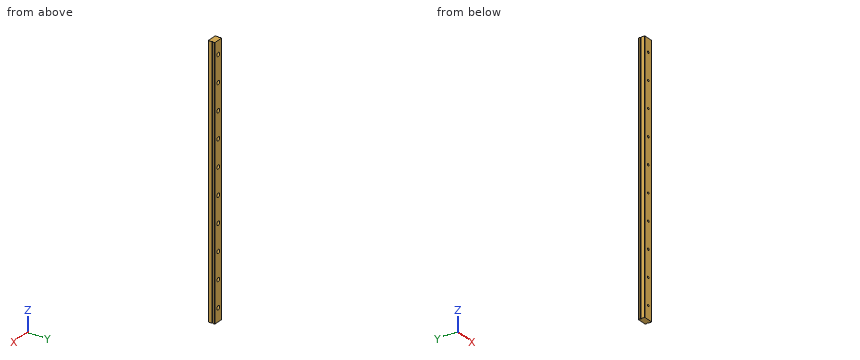
from build123d import *

# Parameters (mm, degrees)
EXTRUDE_1_DEPTH           = 400
HOLE_WIZARD_2_D           = 3.2
HOLE_WIZARD_2_CBORE_D     = 6
HOLE_WIZARD_2_CBORE_DEPTH = 4.5


with BuildPart() as part:
    # 草图1 → 凸台-拉伸1 (new body)
    with BuildSketch(Plane.XY):
        Polygon((-3.269035533, 4.949238579), (10.730964467, 4.949238579), (11.230964467, 4.449238579), (11.230964467, 2.317517259), (10.086764657, 1.783377919), (10.086764657, 0.983377919), (11.230964467, 0.449238579), (11.230964467, -4.550761421), (10.730964467, -5.050761421), (-3.269035533, -5.050761421), (-3.769035533, -4.550761421), (-3.769035533, 0.449238579), (-2.624835723, 0.983377919), (-2.624835723, 1.783377919), (-3.769035533, 2.317517259), (-3.769035533, 4.449238579), align=None)
    extrude(amount=-EXTRUDE_1_DEPTH)

    # 孔2 (through all)
    with Locations(Plane(origin=(3.730964467, 4.949238579, -380), x_dir=(0, 0, 1), z_dir=(0, 1, 0))):
        with Locations((0, 0), (40, 0), (80, 0), (120, 0), (160, 0), (200, 0), (240, 0), (280, 0), (320, 0), (360, 0)):
            CounterBoreHole(HOLE_WIZARD_2_D / 2, HOLE_WIZARD_2_CBORE_D / 2, HOLE_WIZARD_2_CBORE_DEPTH)


solid = part.part
Source: CAD feature listing. Evaluate the final solid. Frame: model axes, mm. Coordinates: 2 decimals unless noted, no trailing zeros. Write each loop counter-clockwise with the first axis right and the second up, starting at its lowest first coordinate (ties: lowest second). Pieces come first, ordered by that corner, then holes. Notation, with made-up numbers: M 81.5,11 L 89.5,11 A26 cw 89.5,33 Z; hole C -34,8.5 d8. An arc over 180 degrees is marked long. Use a Markdown table: item, result.
1) First-contact query: pin 1 Ø2.5 at (x, z) = (3.73, -380) entering from -Y; pin 2 Ø3 at (x, z) = (4.5, -259.5) entering from +Y. Flat tips, straight axial feed; report the tip coordinate or a pass-through.
Conclusion:
| item | result |
|---|---|
| pin 1 | passes through |
| pin 2 | stops at y = 0.45 |
2) Ray query, L1, parallel to X at y = -3.15, z = -380; L2, parallel to X at y = 2.3, z = -60; L3, parallel to X at y = 4.5, z = -248. Return the intervals inside material, ascending.
Conclusion:
| item | result |
|---|---|
| L1 | x = -3.77 to 2.13, 5.33 to 11.23 |
| L2 | x = -3.73 to 0.73, 6.73 to 11.19 |
| L3 | x = -3.72 to 11.18 |
3) Section A-A, the plane z = -166.5. Output: boundary loops of the cut face in (x, y), then the cut area to 3 significant figures.
Conclusion:
| item | result |
|---|---|
| outline | M -3.77,-4.55 L -3.27,-5.05 L 10.73,-5.05 L 11.23,-4.55 L 11.23,0.45 L 10.09,0.98 L 10.09,1.78 L 11.23,2.32 L 11.23,4.45 L 10.73,4.95 L -3.27,4.95 L -3.77,4.45 L -3.77,2.32 L -2.62,1.78 L -2.62,0.98 L -3.77,0.45 Z |
| area | 146 mm^2 |
